from build123d import *

# Parameters (mm, degrees)
SKETCH1_R           = 77.5
BOSS_EXTRUDE1_DEPTH = 22
SKETCH2_R           = 12.5
CUT_EXTRUDE1_DEPTH  = 112.787745303
SKETCH3_R           = 9.094540672
CUT_EXTRUDE2_DEPTH  = 19.915535
CIRPATTERN1_START   = 2.08446524
CIRPATTERN1_DEPTH   = 19.91553476


# Read off the part's stored shape, not the designer's step: CirPattern1
with BuildPart() as part:
    # Sketch1 → Boss-Extrude1 (new body)
    with BuildSketch(Plane(origin=(0, 0, 0), x_dir=(1, 0, 0), z_dir=(0, 1, 0))):
        with Locations(Location((0, 0, 0), (0, 0, 270))):
            Circle(SKETCH1_R)
    extrude(amount=BOSS_EXTRUDE1_DEPTH)

    # Sketch2 → Cut-Extrude1 (cut, through all)
    with BuildSketch(Plane(origin=(0, 0, 0), x_dir=(1, 0, 0), z_dir=(0, 1, 0))):
        with Locations(Location((0, 0, 0), (0, 0, 270))):
            Circle(SKETCH2_R)
    extrude(amount=CUT_EXTRUDE1_DEPTH, mode=Mode.SUBTRACT)

    # Sketch3 → Cut-Extrude2 (cut)
    with BuildSketch(Plane(origin=(0, 22, 0), x_dir=(1, 0, 0), z_dir=(0, 1, 0))):
        with Locations((-16.662496282, 0)):
            Circle(SKETCH3_R)
    extrude(amount=-CUT_EXTRUDE2_DEPTH, mode=Mode.SUBTRACT)

    # CirPattern1 outline → CirPattern1 (cut)
    with BuildSketch(Plane(origin=(0, 0, 0), x_dir=(1, 0, 0), z_dir=(0, 1, 0)).offset(CIRPATTERN1_START)):
        with BuildLine():
            ThreePointArc((-10.537980215, -6.723166886), (-12.913416589, -8.285835594), (-15.655310249, -9.038597586))
            ThreePointArc((-15.655310249, -9.038597586), (-12.878518477, -22.306248328), (0, -18.077195173))
            ThreePointArc((0, -18.077195173), (12.878518477, -22.306248328), (15.655310249, -9.038597586))
            ThreePointArc((15.655310249, -9.038597586), (25.757036954, 0), (15.655310249, 9.038597586))
            ThreePointArc((15.655310249, 9.038597586), (12.878518477, 22.306248328), (0, 18.077195173))
            ThreePointArc((0, 18.077195173), (-12.878518477, 22.306248328), (-15.655310249, 9.038597586))
            ThreePointArc((-15.655310249, 9.038597586), (-12.913416589, 8.285835594), (-10.537980215, 6.723166886))
            ThreePointArc((-10.537980215, 6.723166886), (12.5, 0), (-10.537980215, -6.723166886))
        make_face()
    extrude(amount=CIRPATTERN1_DEPTH, mode=Mode.SUBTRACT)


solid = part.part
The model under review builds one solid part; all positions refer to its coordinate system, in mm. A direction names the side the tool comes from. Round coordinates to 2 decimals unless told otherwise and drop trailing zeros. Loops run counter-clockwise (first coordinate to the right, second up) from the corner with the lowest first, then second, coordinate; pieces in that order, holes last. Notation, with made-up numbers: (19.25, -38.5) -> (29.25, -38.5) arc R11 ccw to (29.25, -34.5) -> close; hole circle Ø7 at (47.5, 49.25). An arc over 180 degrees is marked (long way). One line per question, with ' | ' between items. Start each with the question number.
Item 1: Add section A-A, the plane z = 0. Write out the cut boundary in (x, y).
Item 2: Wall thickness on line 1 along X through (y, z) = (15, 0); line 2 along X through (y, z) = (15.25, -20.5); line 3 along Y through (x, z) = (25, 0): over which ranges is each line inside the solid? List them lowest first. Write a range as [from, to].
Item 3: Machinability: for faces 4 (the face through (12.69, 11.9, 22.41)), 5 (the face through (3.755, 1.028, 11.923)), which of the approach directions +Z, -Z, +X, -X, +Y, -Y give a long, thin tool a straight path to every point of the face, cutting with its end or side? Answer none if there is none.
Item 4: Add section C-C, the plane z = -16. Write out the cut boundary in (x, y), then the cut area to 3 significant figures.
Item 5: For pin 1 (16.5 mm diameter, centred on x = 8.33, z = 14.43, fed in from -Y); pin 2 (12 mm diameter, centred on y = 18, z = 57.5, fed in from -X); pin 3 (2 mm diameter, centred on y = 14.5, z = -6.5, fed in from +X); pin 4 (3 mm diameter, centred on y = 15, z = 1, fed in from +X), all flat-tipped, find the tip position at first contact; note any pin that passes through.
Item 6: Add section B-B, the plane y = 8.5. Write out the cut boundary in (x, z).
Item 7: Draft analysis for pull direction Z (two halves, no side actions). For faces 1 (the face through (-12.69, 11.9, -22.41)), 2 (the face through (-29.68, 10.85, 71.59)), 3 (the face through (18, 22, 16)), state which applies: +Z half, -Z half, draft (parallel to the pull), parting line (faces both ways), or undercut.
Item 8: Add section D-D, the plane x = 59. Write out the cut boundary in (y, z).
Return value:
1) outline: (-77.5, 0) -> (-12.5, 0) -> (-12.5, 2.08) -> (-25.76, 2.08) -> (-25.76, 22) -> (-77.5, 22) -> close; (12.5, 0) -> (77.5, 0) -> (77.5, 22) -> (25.76, 22) -> (25.76, 2.08) -> (12.5, 2.08) -> close
2) line 1: x = [-77.5, -25.76], [25.76, 77.5] | line 2: x = [-74.74, -15.1], [-1.56, 1.56], [15.1, 74.74] | line 3: y = [0, 2.08]
3) face 4: +Y | face 5: +Y, -Y
4) outline: (-75.83, 0) -> (75.83, 0) -> (75.83, 22) -> (17.29, 22) -> (17.29, 2.08) -> (-17.29, 2.08) -> (-17.29, 22) -> (-75.83, 22) -> close | area: 2,650 mm2
5) pin 1: stops at y = 0 | pin 2: stops at x = -57.91 | pin 3: stops at x = 77.3 | pin 4: stops at x = 77.5
6) outline: circle Ø155 at (0, 0); hole (-15.66, -9.04) arc R9.09 ccw (long way) to (0, -18.08) arc R9.09 ccw (long way) to (15.66, -9.04) arc R9.09 ccw (long way) to (15.66, 9.04) arc R9.09 ccw (long way) to (0, 18.08) arc R9.09 ccw (long way) to (-15.66, 9.04) arc R9.09 ccw (long way) to start
7) face 1: undercut | face 2: parting line | face 3: draft
8) outline: (0, -50.25) -> (22, -50.25) -> (22, 50.25) -> (0, 50.25) -> close
